Design review of the part shown in the three views and the two pictorial views. Dimensions are in mm from the part's minimum x, y and z. A direction names the side the tool comes from. Round coordinates to 2 decimals unless told otherwise and drop trailing zeros. Write each loop counter-clockwise with the first axis right and the second up, starting at its lowest first coordinate (ties: lowest second). Pieces come first, ordered by that corner, then holes. Notation, with made-up numbers: (29.5, 45) - (63.5, 45) arc R24 ccw to (63.5, 70) - close; hole circle Ø7 at (0.5, 77). An arc over 180 degrees is marked (long way). Use one line per item in the form item = value.
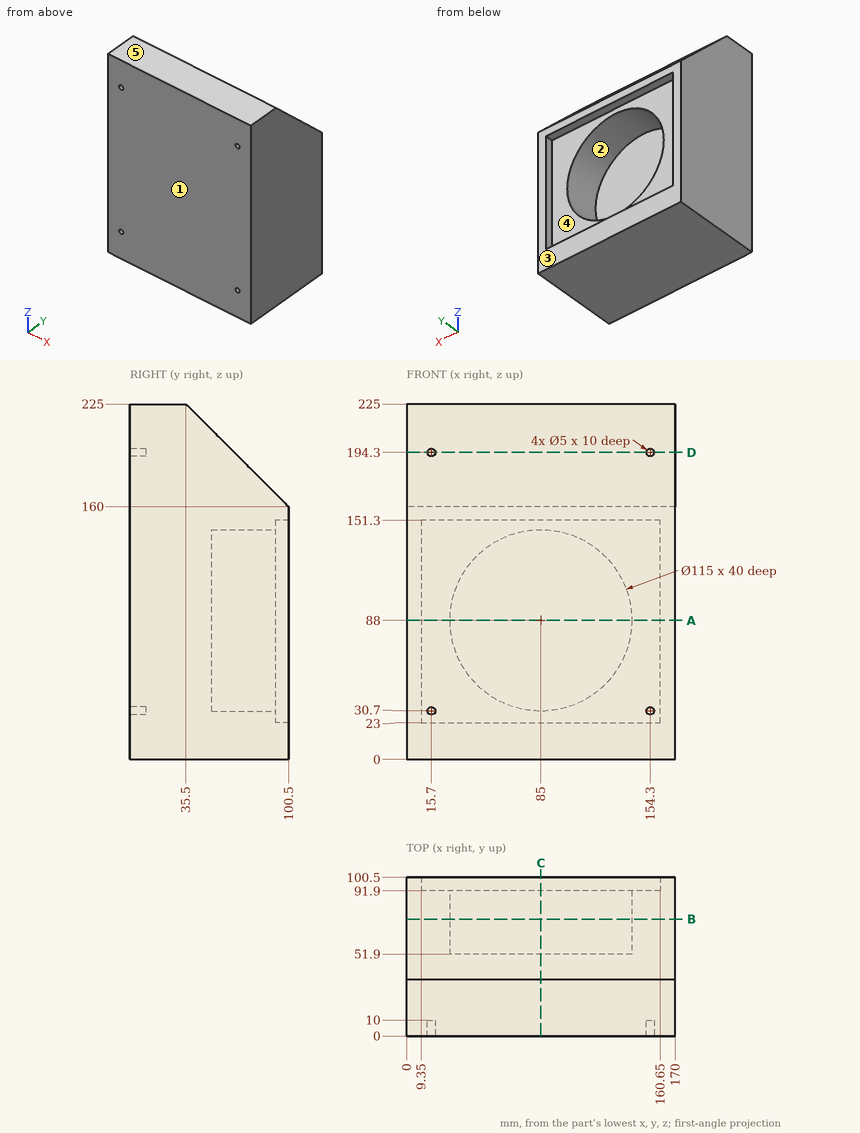
Q1. Draft analysis for pull direction Z (two halves, no side actions). For the marked faces 3, 4 and 5, state which applies: released by +Z, released by -Z, zero draft, split by the parting line, or undercut.
Calculated:
face_3 = zero draft
face_4 = undercut
face_5 = released by +Z
Q2. To check wall thickness, follow line 1 along X through (y, z) = (6, 194.3); line 2 along Z through (x, y) = (15.7, 7.5); line 3 along X through (y, z) = (92.5, 144). State the ranges of each line that lie inside material, in increasing order. Write a range as from..to.
Calculated:
line_1 = 0..13.2, 18.2..151.8, 156.8..170
line_2 = 0..28.2, 33.2..191.8, 196.8..225
line_3 = 0..9.35, 160.65..170
Q3. We need section B-B on y = 74. Write out the cut boundary in (x, z), then the cut area to 3 significant figures.
Calculated:
outline = (0, 0) - (170, 0) - (170, 186.5) - (0, 186.5) - close; hole circle Ø115 at (85, 88)
area = 21,300 mm2
Q4. We need section C-C on x = 85. Write out the cut boundary in (y, z), then the cut area to 3 significant figures.
Calculated:
outline = (0, 0) - (100.5, 0) - (100.5, 23) - (91.9, 23) - (91.9, 30.5) - (51.9, 30.5) - (51.9, 145.5) - (91.9, 145.5) - (91.9, 151.3) - (100.5, 151.3) - (100.5, 160) - (35.5, 225) - (0, 225) - close
area = 14,800 mm2
Q5. We need section D-D on z = 194.3. Write out the cut boundary in (x, y).
Calculated:
outline = (0, 0) - (13.2, 0) - (13.2, 10) - (18.2, 10) - (18.2, 0) - (151.8, 0) - (151.8, 10) - (156.8, 10) - (156.8, 0) - (170, 0) - (170, 66.2) - (0, 66.2) - close
Q6. Machinability: for the marked faces 1 and 2, which of the approach directions +Z, -Z, +X, -X, +Y, -Y give a long, thin tool a straight path to every point of the face, cutting with its end or side? Answer none if there is none.
Calculated:
face_1 = +Z, -Z, +X, -X, -Y
face_2 = +Y
Q7. We need section A-A on z = 88. Write out the cut boundary in (x, y).
Calculated:
outline = (0, 0) - (170, 0) - (170, 100.5) - (160.65, 100.5) - (160.65, 91.9) - (142.5, 91.9) - (142.5, 51.9) - (27.5, 51.9) - (27.5, 91.9) - (9.35, 91.9) - (9.35, 100.5) - (0, 100.5) - close
Q8. For P1, Ø10, axis at y = 66.5, z = 152.5, coming from the -X side; P2, Ø2, axis at x = 101.5, z = 67, coming from the +Y side; P3, Ø9.5, axis at x = 52, y = 97.5, coming from the +Z side; P4, Ø12, axis at x = 32.5, y = 85.5, coming from the +Z side, all flat-tipped, find the tip position at first contact; note any pin that passes through.
Calculated:
P1 = 0
P2 = 51.9
P3 = 167.75
P4 = 181
